```python
from build123d import *

# Parameters (mm, degrees)
SKETCH1_R           = 10
BOSS_EXTRUDE1_DEPTH = 50
SKETCH2_W           = 13
SKETCH2_H           = 2
SKETCH2_W_2         = 20


with BuildPart() as part:
    # Sketch1 → Boss-Extrude1 (new body)
    with BuildSketch(Plane.XY):
        Circle(SKETCH1_R)
    extrude(amount=BOSS_EXTRUDE1_DEPTH)

    # Sketch2 → Cut-Revolve1 (revolve, cut)
    with BuildSketch(Plane(origin=(0, 0, 0), x_dir=(0, 0, -1), z_dir=(1, 0, 0)), mode=Mode.PRIVATE) as cut_revolve1_sk:
        with Locations((-43.5, 9)):
            Rectangle(SKETCH2_W, SKETCH2_H)
        with Locations((-25, 9)):
            Rectangle(SKETCH2_W_2, SKETCH2_H)
        with Locations((-6.5, 9)):
            Rectangle(SKETCH2_W, SKETCH2_H)
    revolve(cut_revolve1_sk.sketch.rotate(Axis((0, 0, 25), (0, 0, -1)), 90), axis=Axis((0, 0, 25), (0, 0, -1)), mode=Mode.SUBTRACT)


solid = part.part
```
Design review of the part built by this model. Coordinates are the model's own, in mm. A direction names the side the tool comes from. Coordinates: 2 decimals unless noted, no trailing zeros. Write each loop counter-clockwise with the first axis right and the second up, starting at its lowest first coordinate (ties: lowest second). Pieces come first, ordered by that corner, then holes. Notation, with made-up numbers: M 53.5,17.5 L 72.5,17.5 A20 cw 72.5,52.5 Z; hole C 4.5,-3 d3. An arc over 180 degrees is marked long. Answer as a JSON object with one key per item and string values.
Item 1: Insertion check: pin 1 Ø5 at (x, y) = (6, 7.5) entering from -Z; pin 2 Ø3 at (x, z) = (-4.5, 27) entering from +Y; pin 3 Ø5 at (x, z) = (3.5, 20) entering from -Y. Each pin has a flat end and moves straight along its axis. Give the tip position at first contact, or say it passes through.
Outcome:
{"pin 1": "z = 0", "pin 2": "y = 7.42", "pin 3": "y = -7.94"}
Item 2: Draft analysis for pull direction Z (two halves, no side actions). For faces 5 (the cylindrical face through (-2.17, -9.76, 35.99)), 6 (the cylindrical face through (-1.73, 7.81, 24.86)), 7 (the flat face through (0, 0, 0)), 8 (the flat face through (0, -8.2, 37)), state which applies: pulls with the +Z half, pulls with the -Z half, needs draft (parallel to the pull), parting line crosses it, or undercut.
Outcome:
{"face 5": "needs draft", "face 6": "undercut", "face 7": "pulls with the -Z half", "face 8": "pulls with the +Z half"}
Item 3: Add section A-A, the plane y = -8.5. Give the boundary of the cut face in (x, z).
Outcome:
{"outline": "M -5.27,13 L 5.27,13 L 5.27,15 L -5.27,15 Z; M -5.27,35 L 5.27,35 L 5.27,37 L -5.27,37 Z"}
Item 4: Wall thickness on probe 1 along Z at (x, y) = (1.75, -9); probe 2 along Y at (x, z) = (6.5, 11.5); probe 3 along Y at (x, z) = (0.5, 16): over which ranges is each line inside the solid? List them lowest first.
Outcome:
{"probe 1": "13 to 15, 35 to 37", "probe 2": "-4.66 to 4.66", "probe 3": "-7.98 to 7.98"}
Item 5: Add section B-B, the plane x = 0. Give the boundary of the cut face in (y, z).
Outcome:
{"outline": "M -10,13 L -8,13 L -8,0 L 8,0 L 8,13 L 10,13 L 10,15 L 8,15 L 8,35 L 10,35 L 10,37 L 8,37 L 8,50 L -8,50 L -8,37 L -10,37 L -10,35 L -8,35 L -8,15 L -10,15 Z"}
Item 6: Machinability: for faces 1 (the flat face through (0, -8.2, 13)), 2 (the cylindrical face through (-2.17, -9.76, 13.99)), 3 (the flat face through (0, -8.2, 35)), 4 (the cylindrical face through (-1.73, 7.81, 43.41)), which of the approach directions +Z, -Z, +X, -X, +Y, -Y give a long, thin tool a straight path to every point of the face, cutting with its end or side? Answer none if there is none.
Outcome:
{"face 1": "-Z", "face 2": "+Z, -Z", "face 3": "none", "face 4": "+Z"}
